Verification items for this drawing (mm, ordinates from the low corner). A direction names the side the tool comes from. Round coordinates to 2 decimals unless told otherwise and drop trailing zeros. Loops run counter-clockwise (first coordinate to the right, second up) from the corner with the lowest first, then second, coordinate; pieces in that order, holes last. Notation, with made-up numbers: (19, -38.5) -> (47, -38.5) arc R17 cw to (47, -34.5) -> close; hole circle Ø2 at (37.5, -25.5). An arc over 180 degrees is marked (long way). One line per question, with ' | ' between items.
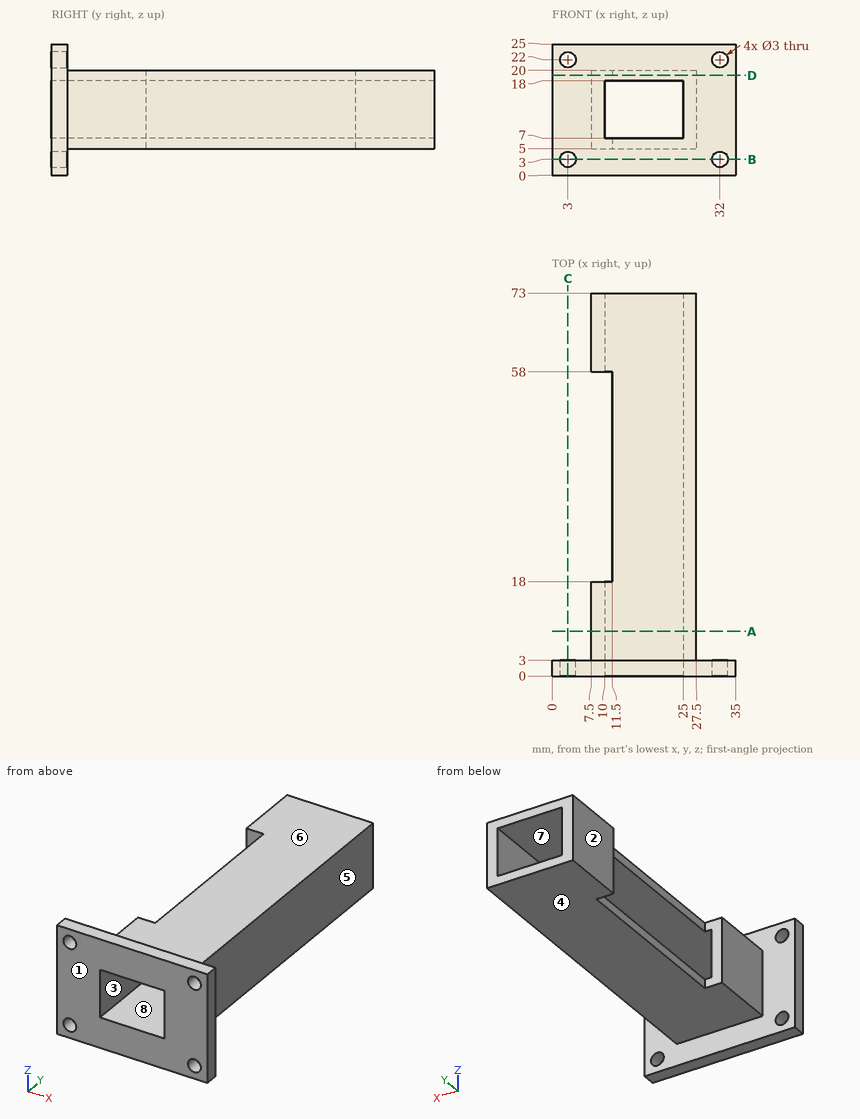
(1) Scan lines: probe 1 along X at (y, z) = (1.3, 3); probe 2 along Z at (x, y) = (14, 4); probe 3 along Z at (x, y) = (8, 15). Record each from-to range of solid material in increasing order.
Answer:
probe 1: x = 0 to 1.5, 4.5 to 30.5, 33.5 to 35 | probe 2: z = 5 to 7, 18 to 20 | probe 3: z = 5 to 20
(2) Mould release check, pull along X, two halves, no side actions. Record for the marked faces 5, 6, 7 and 8: +X half, -X half, draft (parallel to the pull), parting line (faces both ways), or undercut.
Answer:
face 5: +X half | face 6: draft | face 7: undercut | face 8: undercut
(3) Sectioned sample at B-B, the plane z = 3. Record the cut outline in (x, y), and give its area (3 significant figures).
Answer:
outline: (0, 0) -> (1.5, 0) -> (1.5, 3) -> (0, 3) -> close; (4.5, 0) -> (30.5, 0) -> (30.5, 3) -> (4.5, 3) -> close; (33.5, 0) -> (35, 0) -> (35, 3) -> (33.5, 3) -> close | area: 87.0 mm2
(4) Sectioned sample at D-D, the plane z = 19. Record the cut outline in (x, y).
Answer:
outline: (0, 0) -> (35, 0) -> (35, 3) -> (27.5, 3) -> (27.5, 73) -> (7.5, 73) -> (7.5, 58) -> (11.5, 58) -> (11.5, 18) -> (7.5, 18) -> (7.5, 3) -> (0, 3) -> close
(5) Sectioned sample at A-A, the plane y = 8.5. Record the cut outline in (x, z).
Answer:
outline: (7.5, 5) -> (27.5, 5) -> (27.5, 20) -> (7.5, 20) -> close; hole (10, 7) -> (25, 7) -> (25, 18) -> (10, 18) -> close
(6) Sectioned sample at C-C, the plane x = 3. Record the cut outline in (y, z), and give its area (3 significant figures).
Answer:
outline: (0, 0) -> (3, 0) -> (3, 1.5) -> (0, 1.5) -> close; (0, 4.5) -> (3, 4.5) -> (3, 20.5) -> (0, 20.5) -> close; (0, 23.5) -> (3, 23.5) -> (3, 25) -> (0, 25) -> close | area: 57.0 mm2
(7) Go/stop test with flat-tipped pins: pin 1 (7.5 mm diameter, centred on y = 66, z = 12, fed in from -X); pin 2 (7.5 mm diameter, centred on x = 19.5, y = 53.5, fed in from -Z); pin 3 (5 mm diameter, centred on y = 43, z = 4.5, fed in from -X). Record where each tip stops, or that it passes through.
Answer:
pin 1: stops at x = 7.5 | pin 2: stops at z = 5 | pin 3: stops at x = 11.5
(8) Set-up check for the marked faces 1, 2, 3 and 4: record each of +Z, -Z, +X, -X, +Y, -Y from which the full face is reachable in a straight line by a thin tool's end or side.
Answer:
face 1: +Z, -Z, +X, -X, -Y | face 2: +Z, -Z, -X, +Y | face 3: +Y, -Y | face 4: -Z, +X, -X, +Y
